Answer from the drawing. Dimensions are ordinates in mm from the lowest x, y and z of the part. Round coordinates to 2 decimals unless told otherwise and drop trailing zeros. Loops run counter-clockwise (first coordinate to the right, second up) from the corner with the lowest first, then second, coordinate; pieces in that order, holes last. Notation, with made-up numbers: M 37.25,-6.5 L 61.25,-6.5 A18 cw 61.25,28.5 Z; hole C -20.5,23 d7. An arc over 180 degrees is marked long. Answer as a JSON object with one key per item and string values.
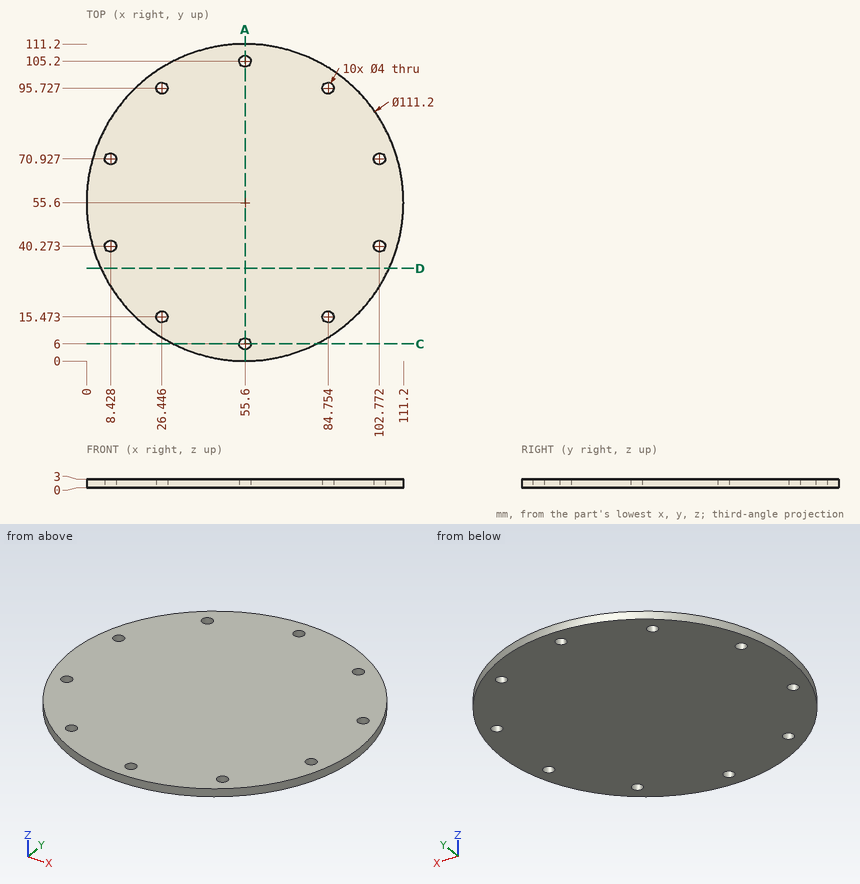
Item 1: The part is cut by section A-A (x = 55.6). Give the vertices of the cut face in (y, z).
Values follow:
{"outline": "M 0,0 L 4,0 L 4,3 L 0,3 Z; M 8,0 L 103.2,0 L 103.2,3 L 8,3 Z; M 107.2,0 L 111.2,0 L 111.2,3 L 107.2,3 Z"}
Item 2: Flat-ended cylindrical pins translate along their axes: P1, Ø5, axis at x = 8.43, y = 40.27, coming from the +Z side; P2, Ø1.5, axis at x = 11.5, z = 1, coming from the +Y side (1 decimal). Find the tip coordinate at first contact, or state that the pin passes through.
Values follow:
{"P1": "z = 3", "P2": "y = 90.4"}
Item 3: The part is cut by section C-C (y = 6). Give the vertices of the cut face in (x, z), then the cut area to 3 significant figures.
Values follow:
{"outline": "M 30.48,0 L 53.6,0 L 53.6,3 L 30.48,3 Z; M 57.6,0 L 80.72,0 L 80.72,3 L 57.6,3 Z", "area": "139 mm^2"}
Item 4: The part is cut by section D-D (y = 32.5). Give the vertices of the cut face in (x, z) (1 decimal).
Values follow:
{"outline": "M 5,0 L 106.2,0 L 106.2,3 L 5,3 Z"}
Item 5: Straight lines are drawn through the part: line 1 (X direction, y = 97, z = 2) (1 decimal); line 2 (X direction, y = 42, z = 2.6) (1 decimal); line 3 (Y direction, x = 56, z = 0.6). For each, find the intervals that lie inside material, in ascending order.
Values follow:
{"line 1": "18.5 to 24.9, 28 to 83.2, 86.3 to 92.7", "line 2": "1.7 to 7.4, 9.4 to 101.8, 103.8 to 109.5", "line 3": "0 to 4.04, 7.96 to 103.24, 107.16 to 111.2"}
